from build123d import *

# Parameters (mm, degrees)
ESBO_O1_R                                            = 6
RESSALTO_EXTRUS_O1_DEPTH                             = 3
REBAIXO_PARA_PARAFUSO_DE_M_QUINA_COM_CAB_D           = 3
REBAIXO_PARA_PARAFUSO_DE_M_QUINA_COM_CAB_CBORE_D     = 5
REBAIXO_PARA_PARAFUSO_DE_M_QUINA_COM_CAB_CBORE_DEPTH = 1.5
ESBO_O3_R                                            = 2
CORTE_EXTRUS_O1_DEPTH                                = 35.715241483


with BuildPart() as part:
    # Esboço1 → Ressalto-extrusão1 (new body)
    with BuildSketch(Plane.XY):
        with BuildLine():
            Line((22.509738768, 13.987877111), (14.731564175, 6.209702518))
            ThreePointArc((14.731564175, 6.209702518), (15.982587719, 0.002329667), (14.727577793, -6.204238442))
            Line((14.727577793, -6.204238442), (22.505752386, -13.982413035))
            ThreePointArc((22.505752386, -13.982413035), (22.734084307, -22.662243955), (14.053133017, -22.48145412))
            Line((14.053133017, -22.48145412), (6.274958424, -14.703279527))
            ThreePointArc((6.274958424, -14.703279527), (0.008088366, -15.99251207), (-6.26285925, -14.723261559))
            Line((-6.26285925, -14.723261559), (-14.041033843, -22.501436152))
            ThreePointArc((-14.041033843, -22.501436152), (-22.526315217, -22.501436152), (-22.526315217, -14.016154778))
            Line((-22.526315217, -14.016154778), (-14.748140624, -6.237980185))
            ThreePointArc((-14.748140624, -6.237980185), (-16.017408692, 0.016872321), (-14.740788367, 6.270228368))
            Line((-14.740788367, 6.270228368), (-22.51896296, 14.048402961))
            ThreePointArc((-22.51896296, 14.048402961), (-22.390928385, 22.410501827), (-14.028587912, 22.521641923))
            Line((-14.028587912, 22.521641923), (-6.250413319, 14.74346733))
            ThreePointArc((-6.250413319, 14.74346733), (0.022005702, 16.007419056), (6.288120931, 14.712577651))
            Line((6.288120931, 14.712577651), (14.066295524, 22.490752244))
            ThreePointArc((14.066295524, 22.490752244), (22.318505349, 22.241631288), (22.509738768, 13.987877111))
        make_face()
        with Locations((-0.017411456, 0.007467609)):
            Circle(ESBO_O1_R, mode=Mode.SUBTRACT)
        with BuildLine():
            ThreePointArc((4.084918003, 12.594218492), (0.002992983, 13.270918226), (-4.088943192, 12.657654219))
            ThreePointArc((-4.088943192, 12.657654219), (-5.733074845, 9.500414621), (-2.575835247, 7.856282968))
            ThreePointArc((-2.575835247, 7.856282968), (-0.036074884, 8.236920288), (2.497471811, 7.816910031))
            ThreePointArc((2.497471811, 7.816910031), (5.679849137, 9.411841166), (4.084918003, 12.594218492))
        make_face(mode=Mode.SUBTRACT)
        with BuildLine():
            ThreePointArc((12.594218492, -4.084918003), (13.270918226, -0.002992983), (12.657654219, 4.088943192))
            ThreePointArc((12.657654219, 4.088943192), (9.500414621, 5.733074845), (7.856282968, 2.575835247))
            ThreePointArc((7.856282968, 2.575835247), (8.236920288, 0.036074884), (7.816910031, -2.497471811))
            ThreePointArc((7.816910031, -2.497471811), (9.411841166, -5.679849137), (12.594218492, -4.084918003))
        make_face(mode=Mode.SUBTRACT)
        with BuildLine():
            ThreePointArc((-4.084918003, -12.594218492), (-0.002992983, -13.270918226), (4.088943192, -12.657654219))
            ThreePointArc((4.088943192, -12.657654219), (5.733074845, -9.500414621), (2.575835247, -7.856282968))
            ThreePointArc((2.575835247, -7.856282968), (0.036074884, -8.236920288), (-2.497471811, -7.816910031))
            ThreePointArc((-2.497471811, -7.816910031), (-5.679849137, -9.411841166), (-4.084918003, -12.594218492))
        make_face(mode=Mode.SUBTRACT)
        with BuildLine():
            ThreePointArc((-12.594218492, 4.084918003), (-13.270918226, 0.002992983), (-12.657654219, -4.088943192))
            ThreePointArc((-12.657654219, -4.088943192), (-9.500414621, -5.733074845), (-7.856282968, -2.575835247))
            ThreePointArc((-7.856282968, -2.575835247), (-8.236920288, -0.036074884), (-7.816910031, 2.497471811))
            ThreePointArc((-7.816910031, 2.497471811), (-9.411841166, 5.679849137), (-12.594218492, 4.084918003))
        make_face(mode=Mode.SUBTRACT)
    extrude(amount=RESSALTO_EXTRUS_O1_DEPTH)

    # Rebaixo para parafuso de máquina com cabeça panela de M22 (through all)
    with Locations(Plane(origin=(8.838834765, 8.838834765, 0), x_dir=(-1, 0, 0), z_dir=(0, 0, -1))):
        with Locations((0, 0), (17.528411311, -0.138256325), (17.67766953, -17.67766953), (0, -17.67766953)):
            CounterBoreHole(REBAIXO_PARA_PARAFUSO_DE_M_QUINA_COM_CAB_D / 2, REBAIXO_PARA_PARAFUSO_DE_M_QUINA_COM_CAB_CBORE_D / 2, REBAIXO_PARA_PARAFUSO_DE_M_QUINA_COM_CAB_CBORE_DEPTH)

    # Esboço3 → Corte-extrusão1 (cut, through all)
    with BuildSketch(Plane(origin=(0, 0, 0), x_dir=(-1, 0, 0), z_dir=(0, 0, -1))):
        with Locations((-18.285022442, 18.273775436)):
            Circle(ESBO_O3_R)
        with Locations((18.273775436, 18.285022442)):
            Circle(ESBO_O3_R)
        with Locations((18.285022442, -18.273775436)):
            Circle(ESBO_O3_R)
        with Locations((-18.273775436, -18.285022442)):
            Circle(ESBO_O3_R)
    extrude(amount=-CORTE_EXTRUS_O1_DEPTH, mode=Mode.SUBTRACT)


solid = part.part
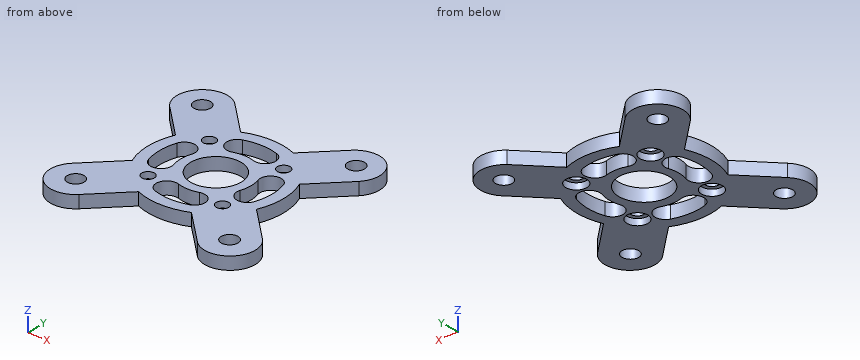
CAD build for the part. Positions are in the model's coordinates, mm. Round coordinates to 2 decimals unless told otherwise and drop trailing zeros. Write each loop counter-clockwise with the first axis right and the second up, starting at its lowest first coordinate (ties: lowest second). Pieces come first, ordered by that corner, then holes. Notation, with made-up numbers: (26, -20) -> (76, -20) arc R28 ccw to (76, 9) -> close; hole circle Ø5 at (17, 13). An arc over 180 degrees is marked (long way). Answer as a JSON object with one key per item and string values.
(1) Band-saw the part on B-B, the plane z = 0.6. Count the separate pieces of the cut face and the enclosed holes in it, then the cut area to 3 significant figures.
Reported:
{"separate pieces": "1", "enclosed holes": "13", "area": "1,060 mm^2"}
(2) Band-saw the part on C-C, the plane x = -5. List the corners of the cut face in (y, z), then the cut area to 3 significant figures.
Reported:
{"outline": "(-15.2, 0) -> (-12.05, 0) -> (-12.05, 3) -> (-15.2, 3) -> close; (-8.36, 0) -> (-3.34, 0) -> (-3.34, 3) -> (-8.36, 3) -> close; (3.35, 0) -> (8.37, 0) -> (8.37, 3) -> (3.35, 3) -> close; (12.14, 0) -> (15.21, 0) -> (15.21, 3) -> (12.14, 3) -> close", "area": "48.8 mm^2"}
(3) Pin check, flat tips, straight feed: P1, Ø1.5, axis at y = 16, z = 2, coming from the +X side; P2, Ø4.5, axis at x = 8.84, y = -8.84, coming from the -Z side; P3, Ø1.5, axis at y = 8.5, z = 1.5, coming from the +X side. Stop position of each tip, or through.
Reported:
{"P1": "stops at x = 23.93", "P2": "stops at z = 1.5", "P3": "stops at x = 17.77"}
(4) Band-saw the part on A-A, the plane x = -18.5. List the corners of the cut face in (y, z), then the cut area to 3 significant figures.
Reported:
{"outline": "(-24.25, 0) -> (-20.26, 0) -> (-20.26, 3) -> (-24.25, 3) -> close; (-16.29, 0) -> (-9.99, 0) -> (-9.99, 3) -> (-16.29, 3) -> close; (10.03, 0) -> (16.3, 0) -> (16.3, 3) -> (10.03, 3) -> close; (20.27, 0) -> (24.15, 0) -> (24.15, 3) -> (20.27, 3) -> close", "area": "61.3 mm^2"}
(5) Probe probe 1 along Y at (x, z) = (-2.5, 0.75); probe 2 along Y at (x, z) = (1.5, 1.45); probe 3 along X at (y, z) = (3, 0.45). List the from-to ranges inside material, lowest first. Write a range as [from, to].
Reported:
{"probe 1": "y = [-15.8, -13.01], [-7.82, -5.45], [5.47, 7.88], [13.05, 15.81]", "probe 2": "y = [-15.92, -13.2], [-8.12, -5.8], [5.81, 8.08], [13.17, 15.94]", "probe 3": "x = [-15.74, -12.9], [-7.71, -5.22], [5.18, 7.76], [12.95, 15.7]"}
